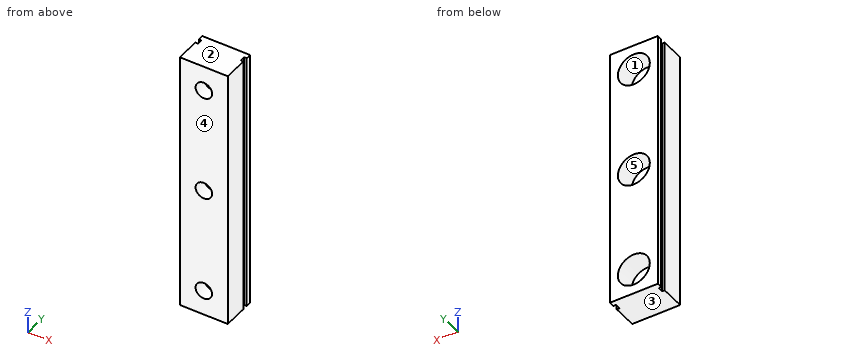
```python
from build123d import *

# Parameters (mm, degrees)
SKETCH_1_W          = 9
SKETCH_1_H          = 49.5
EXTRUDE_1_DEPTH     = 6.5
SKETCH_2_R          = 1.55
CUT_EXTRUDE_1_DEPTH = 51.729675733
SKETCH_3_R          = 3
CUT_EXTRUDE_2_DEPTH = 4
SKETCH_4_W          = 0.5
SKETCH_4_H          = 1
CUT_EXTRUDE_3_DEPTH = 51.729675733


with BuildPart() as part:
    # 草图1 → 凸台-拉伸1 (new body)
    with BuildSketch(Plane(origin=(0, 0, 0), x_dir=(1, 0, 0), z_dir=(0, 1, 0))):
        with Locations((4.5, -24.75)):
            Rectangle(SKETCH_1_W, SKETCH_1_H)
    extrude(amount=EXTRUDE_1_DEPTH)

    # 草图2 → 切除-拉伸1 (cut, through all)
    with BuildSketch(Plane(origin=(0, 6.5, 0), x_dir=(1, 0, 0), z_dir=(0, 1, 0))):
        with Locations(Location((4.5, -24.75, 0), (0, 0, 270))):
            Circle(SKETCH_2_R)
        with Locations(Location((4.5, -4.75, 0), (0, 0, 270))):
            Circle(SKETCH_2_R)
        with Locations(Location((4.5, -44.75, 0), (0, 0, 270))):
            Circle(SKETCH_2_R)
    extrude(amount=-CUT_EXTRUDE_1_DEPTH, mode=Mode.SUBTRACT)

    # 草图3 → 切除-拉伸2 (cut)
    with BuildSketch(Plane(origin=(0, 6.5, 0), x_dir=(1, 0, 0), z_dir=(0, 1, 0))):
        with Locations(Location((4.5, -44.75, 0), (0, 0, 270))):
            Circle(SKETCH_3_R)
        with Locations(Location((4.5, -24.75, 0), (0, 0, 270))):
            Circle(SKETCH_3_R)
        with Locations(Location((4.5, -4.75, 0), (0, 0, 270))):
            Circle(SKETCH_3_R)
    extrude(amount=-CUT_EXTRUDE_2_DEPTH, mode=Mode.SUBTRACT)

    # 草图4 → 切除-拉伸3 (cut, through all)
    with BuildSketch(Plane.XY.offset(49.5)):
        with Locations((0.25, 5)):
            Rectangle(SKETCH_4_W, SKETCH_4_H)
        with Locations((8.75, 5)):
            Rectangle(SKETCH_4_W, SKETCH_4_H)
    extrude(amount=-CUT_EXTRUDE_3_DEPTH, mode=Mode.SUBTRACT)


solid = part.part
```
Design review of the part built by this model. Coordinates are the model's own, in mm. Face numbers are marked on the shaded views. A direction names the side the tool comes from. Give positions to 0.01 mm unless a question says otherwise; leave off trailing zeros. Write each loop counter-clockwise with the first axis right and the second up, starting at its lowest first coordinate (ties: lowest second). Pieces come first, ordered by that corner, then holes. Notation, with made-up numbers: (9, 48) - (54, 48) arc R14 ccw to (54, 69) - close; hole circle Ø11 at (12.5, 70.5). An arc over 180 degrees is marked (long way). Return JSON: item names as keys, results as strings. Group by question number.
(1) We need section C-C, the plane y = 1.25. Give the boundary of the cut face in (x, z), then the cut area to 3 significant figures.
(2) Mouldability with a two-part tool opening along Z and no side actions: class the marked faces 3, 4 and 5 as +Z half, -Z half, draft (parallel to the pull), parting line (faces both ways), or undercut.
(3) To check wall thickness, follow probe 1 along X at (y, z) = (5.75, 25); probe 2 along Z at (x, y) = (3.25, 4); probe 3 along Z at (x, y) = (5.5, 4). State the ranges of each line that lie inside material, in increasing order.
(4) We need section D-D, the plane z = 11. Give the boundary of the cut face in (x, y), then the cut area to 3 significant figures.
(5) We need section B-B, the plane x = 4.5. Give the boundary of the cut face in (y, z), then the cut area to 4 significant figures.
(6) Insertion check: pin 1 (5 mm diameter, centred on x = 4.5, z = 24.75, fed in from +Y); pin 2 (0.8 mm diameter, centred on y = 5, z = 15, fed in from +X). Each pin has a flat end and moves straight along its axis. Give the tip position at first contact, or say it passes through.
(7) Machinability: for the marked faces 1 and 2, which of the approach directions +Z, -Z, +X, -X, +Y, -Y give a long, thin tool a straight path to every point of the face, cutting with its end or side? Answer none if there is none.
(8) We need section A-A, the plane z = 24.75. Give the boundary of the cut face in (x, y).
Reported:
{
 "1": {"outline": "(0, 0) - (9, 0) - (9, 49.5) - (0, 49.5) - close; hole circle Ø3.1 at (4.5, 4.75); hole circle Ø3.1 at (4.5, 24.75); hole circle Ø3.1 at (4.5, 44.75)", "area": "423 mm2"},
 "2": {"face 3": "-Z half", "face 4": "draft", "face 5": "undercut"},
 "3": {"probe 1": "x = 0 to 1.51, 7.49 to 9", "probe 2": "z = 0 to 2.02, 7.48 to 22.02, 27.48 to 42.02, 47.48 to 49.5", "probe 3": "z = 0 to 1.92, 7.58 to 21.92, 27.58 to 41.92, 47.58 to 49.5"},
 "4": {"outline": "(0, 0) - (9, 0) - (9, 4.5) - (8.5, 4.5) - (8.5, 5.5) - (9, 5.5) - (9, 6.5) - (0, 6.5) - (0, 5.5) - (0.5, 5.5) - (0.5, 4.5) - (0, 4.5) - close", "area": "57.5 mm2"},
 "5": {"outline": "(0, 0) - (6.5, 0) - (6.5, 1.75) - (2.5, 1.75) - (2.5, 3.2) - (0, 3.2) - close; (0, 6.3) - (2.5, 6.3) - (2.5, 7.75) - (6.5, 7.75) - (6.5, 21.75) - (2.5, 21.75) - (2.5, 23.2) - (0, 23.2) - close; (0, 26.3) - (2.5, 26.3) - (2.5, 27.75) - (6.5, 27.75) - (6.5, 41.75) - (2.5, 41.75) - (2.5, 43.2) - (0, 43.2) - close; (0, 46.3) - (2.5, 46.3) - (2.5, 47.75) - (6.5, 47.75) - (6.5, 49.5) - (0, 49.5) - close", "area": "226.5 mm2"},
 "6": {"pin 1": "stops at y = 2.5", "pin 2": "stops at x = 8.5"},
 "7": {"face 1": "+Y", "face 2": "+Z, +X, -X, +Y, -Y"},
 "8": {"outline": "(0, 0) - (2.95, 0) - (2.95, 2.5) - (1.5, 2.5) - (1.5, 6.5) - (0, 6.5) - (0, 5.5) - (0.5, 5.5) - (0.5, 4.5) - (0, 4.5) - close; (6.05, 0) - (9, 0) - (9, 4.5) - (8.5, 4.5) - (8.5, 5.5) - (9, 5.5) - (9, 6.5) - (7.5, 6.5) - (7.5, 2.5) - (6.05, 2.5) - close"}
}
